```python
from build123d import *

# Parameters (mm, degrees)
SKETCH1_W           = 20
SKETCH1_H           = 10
BOSS_EXTRUDE1_DEPTH = 1
SKETCH2_W           = 12
SKETCH2_H           = 6.5
CUT_EXTRUDE1_DEPTH  = 4
SKETCH3_R           = 1
BOSS_EXTRUDE2_DEPTH = 1


with BuildPart() as part:
    # Sketch1 → Boss-Extrude1 (new body)
    with BuildSketch(Plane(origin=(0, 0, 0), x_dir=(1, 0, 0), z_dir=(0, 1, 0))):
        Rectangle(SKETCH1_W, SKETCH1_H)
    extrude(amount=BOSS_EXTRUDE1_DEPTH)

    # Sketch2 → Cut-Extrude1 (cut)
    with BuildSketch(Plane(origin=(0, 1, 0), x_dir=(1, 0, 0), z_dir=(0, 1, 0))):
        Rectangle(SKETCH2_W, SKETCH2_H)
    extrude(amount=-CUT_EXTRUDE1_DEPTH, mode=Mode.SUBTRACT)

    # Sketch3 → Boss-Extrude2 (add)
    with BuildSketch(Plane(origin=(0, 1, 0), x_dir=(1, 0, 0), z_dir=(0, 1, 0))):
        with Locations(Location((-7.7, 0, 0), (0, 0, 90))):
            Circle(SKETCH3_R)
        with Locations(Location((7.7, 0, 0), (0, 0, 90))):
            Circle(SKETCH3_R)
    extrude(amount=BOSS_EXTRUDE2_DEPTH)


solid = part.part
```
Check sheet for the modelled part. Datum: model origin and axes. Units: mm. A direction names the side the tool comes from. Round coordinates to 2 decimals unless told otherwise and drop trailing zeros. Loops run counter-clockwise (first coordinate to the right, second up) from the corner with the lowest first, then second, coordinate; pieces in that order, holes last. Notation, with made-up numbers: (45, 41.25) - (50, 41.25) arc R29 ccw to (50, 75.25) - close; hole circle Ø3 at (-22.75, 80.5). An arc over 180 degrees is marked (long way). Write item = value, one per line. Start each with the question number.
Q1. Thickness scan on L1, parallel to X at y = 0.7, z = 0; L2, parallel to Z at x = 2.25, y = 0.55; L3, parallel to X at y = 1.45, z = 0. Record the ranges inside material, lowest first.
Q2. Release check for a two-part mould opening along Z. For faces 4 (the face through (-0.1, 0.5, -3.25)), 5 (the face through (-10, 0.5, 0.1)), 6 (the face through (-0.1, 0.5, 3.25)), 7 (the face through (-0.1, 0.5, 5)) record: pulls with the +Z half, pulls with the -Z half, needs draft (parallel to the pull), parting line crosses it, or undercut.
Q3. Section check C-C (y = 0.2). Record the boundary of the cut face in (x, z), plus the area to 3 significant figures.
Q4. Section check B-B (z = 2.5). Record the boundary of the cut face in (x, y).
Q5. Depth check by flat-ended pin: P1, Ø3, axis at x = 4.5, z = -3, coming from the -Y side. Enter the tip coordinate at first touch or a pass-through.
Q6. Section check A-A (x = 2.75). Record the boundary of the cut face in (y, z).
Q7. Section check D-D (y = 1.8). Record the boundary of the cut face in (x, z).
Q8. Access from +Z, -Z, +X, -X, +Y, -Y to the whole of each face (thin tool, end or side, straight path). Record for faces 1 (the face through (6, 0.5, 0)), 2 (the face through (8.3, 1.5, 0.8)), 3 (the face through (10, 0.5, 0.1)).
Derived:
q1.L1 = -10 to -6, 6 to 10
q1.L2 = -5 to -3.25, 3.25 to 5
q1.L3 = -8.7 to -6.7, 6.7 to 8.7
q2.face_4 = undercut
q2.face_5 = needs draft
q2.face_6 = undercut
q2.face_7 = pulls with the +Z half
q3.outline = (-10, -5) - (10, -5) - (10, 5) - (-10, 5) - close; hole (-6, -3.25) - (6, -3.25) - (6, 3.25) - (-6, 3.25) - close
q3.area = 122 mm^2
q4.outline = (-10, 0) - (-6, 0) - (-6, 1) - (-10, 1) - close; (6, 0) - (10, 0) - (10, 1) - (6, 1) - close
q5.P1 = 0
q6.outline = (0, -5) - (1, -5) - (1, -3.25) - (0, -3.25) - close; (0, 3.25) - (1, 3.25) - (1, 5) - (0, 5) - close
q7.outline = circle Ø2 at (-7.7, 0); circle Ø2 at (7.7, 0)
q8.face_1 = +Y, -Y
q8.face_2 = +Y
q8.face_3 = +Z, -Z, +X, +Y, -Y
